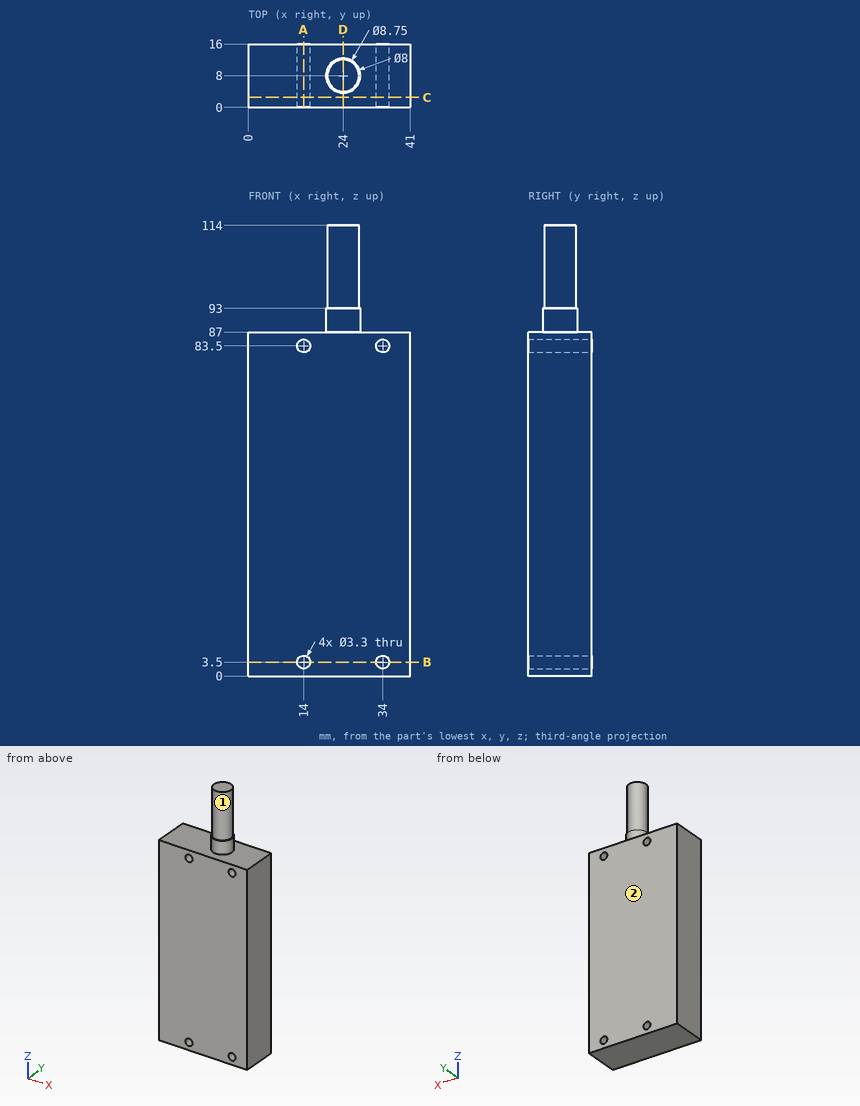
Verification items for this drawing (mm, ordinates from the low corner). A direction names the side the tool comes from. Coordinates: 2 decimals unless noted, no trailing zeros. Write each loop counter-clockwise with the first axis right and the second up, starting at its lowest first coordinate (ties: lowest second). Pieces come first, ordered by that corner, then holes. Notation, with made-up numbers: M 88,-23 L 94,-23 A26 ccw 94,-1 Z; hole C 56.25,50 d3. An arc over 180 degrees is marked long. One line per item, written item: value. Start each with the question number.
(1) Scan lines: line 1 along X through (y, z) = (8.5, 83.5); line 2 along Z through (x, y) = (14, 7); line 3 along Z through (x, y) = (33, 12.25). Record each from-to range of solid material in increasing order. Write a range as [from, to].
(2) Tool access check on the marked faces 1 and 2. Record the directions out of +Z, -Z, +X, -X, +Y, -Y that give a thin tool (end or side, any length) a straight path to the whole face; none if there is none.
(3) Depth check by flat-ended pin: pin 1 (6 mm diameter, centred on x = 33, y = 9.5, fed in from +Z). Enter the tip coordinate at first touch or a pass-through.
(4) Sectioned sample at D-D, the plane x = 24. Enter the section's corners in (y, z) (3 decimals), and give its area (3 significant figures).
(5) Sectioned sample at C-C, the plane y = 2.5. Enter the section's corners in (x, z).
(6) Sectioned sample at B-B, the plane z = 3.5. Enter the section's corners in (x, y), and give its area (3 significant figures).
(7) Sectioned sample at A-A, the plane x = 14. Enter the section's corners in (y, z), and give its area (3 significant figures).
Filled sheet:
1. line 1: [0, 12.35], [15.65, 32.35], [35.65, 41]
1. line 2: [0, 1.85], [5.15, 81.85], [85.15, 87]
1. line 3: [0, 2.19], [4.81, 82.19], [84.81, 87]
2. face 1: +Z
2. face 2: +Z, -Z, +X, -X, +Y
3. pin 1: z = 87
4. outline: M 0,0 L 16,0 L 16,87 L 12.375,87 L 12.375,93 L 12,93 L 12,114 L 4,114 L 4,93 L 3.625,93 L 3.625,87 L 0,87 Z
4. area: 1,610 mm²
5. outline: M 0,0 L 41,0 L 41,87 L 0,87 Z; hole C 14,3.5 d3.3; hole C 14,83.5 d3.3; hole C 34,3.5 d3.3; hole C 34,83.5 d3.3
6. outline: M 0,0 L 12.35,0 L 12.35,16 L 0,16 Z; M 15.65,0 L 32.35,0 L 32.35,16 L 15.65,16 Z; M 35.65,0 L 41,0 L 41,16 L 35.65,16 Z
6. area: 550 mm²
7. outline: M 0,0 L 16,0 L 16,1.85 L 0,1.85 Z; M 0,5.15 L 16,5.15 L 16,81.85 L 0,81.85 Z; M 0,85.15 L 16,85.15 L 16,87 L 0,87 Z
7. area: 1,290 mm²
